Check sheet for the modelled part. Datum: model origin and axes. Units: mm. Face numbers are marked on the shaded views. A direction names the side the tool comes from. Round coordinates to 2 decimals unless told otherwise and drop trailing zeros. Order: outer loops, then holes, each group sorted by start corner. A loop starts at its lowest first (then second) coordinate and runs counter-clockwise, first axis right, second up. Notation, with made-up numbers: (67.25, 30) -> (111.25, 30) arc R20 cw to (111.25, 53) -> close; hole circle Ø6 at (11, 14.5). An arc over 180 degrees is marked (long way). Use CSV: the item, a comma, the result in double quotes.
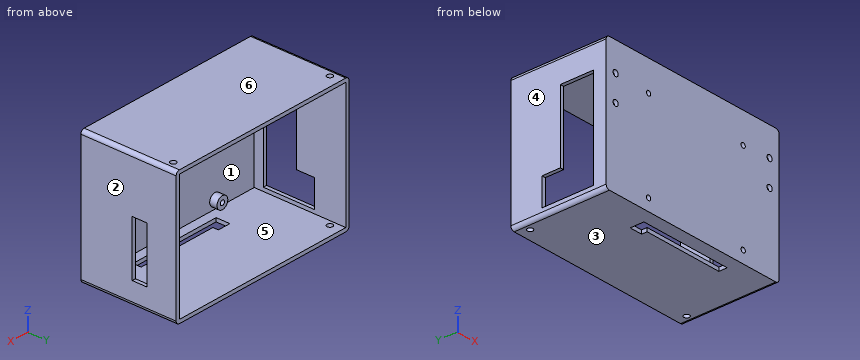
Autodesk Inventor part; units mm, degrees
ref_plane "YZ Plane" through (0, 0, 0) normal (1, 0, 0) x (0, 1, 0)
ref_plane "XZ Plane" through (0, 0, 0) normal (0, 1, 0) x (-1, 0, 0)
ref_plane "XY Plane" through (0, 0, 0) normal (0, 0, 1) x (1, 0, 0)
sketch "Náčrt1" plane through (0, 0, 0) normal (0, 1, 0) x (-1, 0, 0)
  line L0 (0, 0) -> (-106, 0)
  line L1 (-106, 0) -> (-106, -62)
  line L2 (-106, -62) -> (0, -62)
  line L3 (0, -62) -> (0, 0)
  line L4 (-104, -2) -> (-2, -2)
  line L5 (-2, -2) -> (-2, -60)
  line L6 (-2, -60) -> (-104, -60)
  line L7 (-104, -60) -> (-104, -2)
  line L8 (-5.8, 0) -> (-5.8, -18) construction
  circle A0 centre (-5.8, -19.6) radius 1.6
  line L9 (0, -19.6) -> (-4.2, -19.6) construction
  line L10 (-7.4, 0) -> (-7.4, -5.6) construction
  circle A1 centre (-5.8, -5.6) radius 1.6
  line L11 (0, -7.2) -> (-5.8, -7.2) construction
  line L12 (-53, 11.0609) -> (-53, -73.3805) construction
  line L13 (-100.2, 0) -> (-100.2, -18) construction
  circle A2 centre (-100.2, -19.6) radius 1.6
  line L14 (-106, -19.6) -> (-101.8, -19.6) construction
  line L15 (-98.6, 0) -> (-98.6, -5.6) construction
  circle A3 centre (-100.2, -5.6) radius 1.6
  line L16 (-106, -7.2) -> (-100.2, -7.2) construction
  dimension "d0" = 62
  dimension "d1" = 106
  dimension "d2" = 2
  dimension "d8" = 18
  dimension "d9" = 4.2
  dimension "d10" = 3.2
  dimension "d13" = 5.8
  dimension "d14" = 5.6
  dimension "d15" = 3.2
extrude "Vysunutí1" add sketch "Náčrt1" along normal blind 2 contours L4 L5 L6 L7 | A0 | A1 | A2 | A3
extrude "Vysunutí2" add sketch "Náčrt1" along normal blind 52 contours L3 L2 L1 L0
extrude "Vysunutí3" cut sketch "Náčrt1" along normal blind 2 contours A0 | A1 | A2 | A3
sketch "Náčrt2" plane through (0, 2, 0) normal (0, 1, 0) x (1, 0, 0)
  circle A0 centre (84, 55.5) radius 1.3
  line L0 (2, 60) -> (104, 60)
  circle A1 centre (26, 55.5) radius 1.3
  line L1 (2, 2) -> (2, 60)
  circle A2 centre (26, 6.5) radius 1.3
  circle A3 centre (84, 6.5) radius 1.3
  line L2 (104, 2) -> (2, 2)
  circle A4 centre (26, 6.5) radius 3.3
  circle A5 centre (26, 55.5) radius 3.3
  circle A6 centre (84, 55.5) radius 3.3
  circle A7 centre (84, 6.5) radius 3.3
  point P0 (0, 0)
  dimension "d19" = 4.5
  dimension "d20" = 2.6
  dimension "d21" = 2.6
  dimension "d22" = 58
  dimension "d23" = 24
  dimension "d24" = 4.5
  dimension "d25" = 2.6
  dimension "d26" = 24
  dimension "d27" = 2.6
  dimension "d28" = 58
  dimension "d29" = 4.5
  dimension "d30" = 4.5
  dimension "d31" = 49
  dimension "d32" = 2
  dimension "d33" = 2
  dimension "d34" = 2
  dimension "d35" = 2
extrude "Vysunutí4" add sketch "Náčrt2" along normal blind 4
extrude "Vysunutí5" cut sketch "Náčrt2" against normal blind 2 contours A0 | A1 | A2 | A3
sketch "Náčrt3" plane through (0, 0, -62) normal (-1, 0, 0) x (0, 0, 1)
  line L0 (4, 7) -> (58, 7)
  line L1 (58, 7) -> (58, 25)
  line L2 (58, 25) -> (4, 25)
  line L3 (4, 25) -> (4, 7)
  line L4 (9.8, 6) -> (3.2, 6)
  line L5 (2, 2) -> (2, 52)
  line L6 (60, 2) -> (60, 52)
  point P0 (62, 0)
  dimension "d40" = 1
  dimension "d41" = 54
  dimension "d42" = 18
  dimension "d43" = 2
  dimension "d44" = 2
extrude "Vysunutí6" cut sketch "Náčrt3" against normal blind 2
sketch "Náčrt4" plane through (106, 0, -62) normal (0, 0, -1) x (-1, 0, 0)
  line L0 (24, 7) -> (75, 7)
  line L1 (75, 7) -> (75, 11.5)
  line L2 (75, 11.5) -> (24, 11.5)
  line L3 (24, 11.5) -> (24, 7)
  line L4 (104, 2) -> (104, 52)
  line L5 (75, 11.5) -> (68, 11.5)
  line L6 (68, 11.5) -> (68, 14.5)
  line L7 (68, 14.5) -> (75, 14.5)
  line L8 (75, 14.5) -> (75, 11.5)
  line L9 (2, 2) -> (104, 2)
  point P0 (106, 0)
  point P1 (68, 11.5)
  dimension "d47" = 4.5
  dimension "d48" = 29
  dimension "d49" = 51
  dimension "d50" = 5
  dimension "d51" = 7.5
  dimension "d52" = 7
extrude "Vysunutí7" cut sketch "Náčrt4" against normal blind 2
sketch "Náčrt5" plane through (0, 0, 0) normal (0, -1, 0) x (1, 0, 0)
  line L0 (106, 0) -> (106, -62)
  line L1 (106, -2) -> (0, -2)
  line L2 (0, -2) -> (0, 10)
  line L3 (0, 10) -> (106, 10)
  line L4 (106, 10) -> (106, -2)
  line L5 (2, -2) -> (104, -2)
  line L6 (106, 10) -> (0, 10)
  line L7 (0, 10) -> (0, 8)
  line L8 (0, 8) -> (106, 8)
  line L9 (106, 8) -> (106, 10)
  line L10 (104, -60) -> (104, -2)
  line L11 (104, -2) -> (106, -2)
  line L12 (106, -2) -> (106, 10)
  line L13 (106, 10) -> (104, 10)
  line L14 (104, 10) -> (104, -2)
  line L15 (2, -2) -> (2, -60)
  line L16 (2, -2) -> (0, -2)
  line L17 (0, -2) -> (0, 10)
  line L18 (0, 10) -> (2, 10)
  line L19 (2, 10) -> (2, -2)
  point P0 (0, 0)
  point P1 (2, 8)
  point P2 (104, 8)
  dimension "d55" = 12
  dimension "d56" = 106
  dimension "d57" = 2
extrude "Vysunutí8" cut sketch "Náčrt5" against normal blind 52 contours L1 L19 L8 L14
extrude "Vysunutí9" add sketch "Náčrt5" against normal blind 2 contours L1 L19 L8 L14
extrude "Vysunutí10" add sketch "Náčrt5" against normal blind 52 contours L0 L1 L14 L8 L4 | L8 L14 L3 L4 | L8 L19 L3 L14 | L1 L2 L8 L19 | L8 L2 L3 L19
sketch "Náčrt6" plane through (0, 0, -62) normal (-1, 0, 0) x (0, 0, 1)
  line L0 (4, 25) -> (58, 25)
  line L1 (4, 25) -> (19, 25)
  line L2 (19, 25) -> (19, 35)
  line L3 (19, 35) -> (4, 35)
  line L4 (4, 35) -> (4, 25)
  point P0 (62, 0)
  dimension "d64" = 15
  dimension "d65" = 10
extrude "Vysunutí11" cut sketch "Náčrt6" against normal blind 4
fillet "Zaoblení1" radius 2 4 edges at (106, 26, -62) (0, 26, -62) (0, 26, 10) (106, 26, 10)
sketch "Náčrt7" plane through (2, 0, 10) normal (0, 0, 1) x (1, 0, 0)
  circle A0 centre (3, 46) radius 1.55
  line L0 (0, 52) -> (102, 52)
  line L1 (0, 0) -> (0, 52)
  circle A1 centre (99, 46) radius 1.55
  line L2 (102, 52) -> (102, 0)
  point P0 (-2, 0)
  dimension "d69" = 3.1
  dimension "d70" = 6
  dimension "d71" = 3
  dimension "d72" = 3.1
  dimension "d73" = 3
  dimension "d74" = 6
extrude "Vysunutí12" cut sketch "Náčrt7" against normal blind 400
sketch "Náčrt8" plane through (106, 0, 8) normal (1, 0, 0) x (0, 0, -1)
  line L0 (28, 36) -> (58, 36)
  line L1 (58, 36) -> (58, 28)
  line L2 (58, 28) -> (28, 28)
  line L3 (28, 28) -> (28, 36)
  line L4 (70, 0) -> (70, 52)
  line L5 (0, 0) -> (68, 0)
  point P0 (8, 0)
  dimension "d77" = 12
  dimension "d78" = 30
  dimension "d79" = 8
  dimension "d80" = 28
extrude "Vysunutí13" cut sketch "Náčrt8" against normal blind 52
equation "\"d21\" = d20"
equation "\"d24\" = d19"
equation "\"d25\" = d20"
equation "\"d26\" = d23"
equation "\"d27\" = d20"
equation "\"d28\" = d22"
equation "\"d29\" = d19"
equation "\"d30\" = d19"
equation "\"d33\" = d32"
equation "\"d34\" = d32"
equation "\"d35\" = d32"
properties part number "RPIholder"
Q1. Go/stop test with flat-tipped pins: pin 1 (3.5 mm diameter, centred on x = 5.8, z = -5.6, fed in from +Y); pin 2 (1.6 mm diameter, centred on x = 105, z = -34.5, fed in from -Y); pin 3 (5.5 mm diameter, centred on x = 27, z = -7.5, fed in from +Y). Record where each tip stops, or that it passes through.
Result sheet:
pin 1,"stops at y = 2"
pin 2,"stops at y = 0"
pin 3,"stops at y = 6"
Q2. Sectioned sample at C-C, the plane x = 77.5. Enter the section's corners in (y, z).
Result sheet:
outline,"(0, -62) -> (7, -62) -> (7, -60) -> (2, -60) -> (2, 8) -> (52, 8) -> (52, 10) -> (0, 10) -> close; (11.5, -62) -> (52, -62) -> (52, -60) -> (11.5, -60) -> close"
Q3. Access from +Z, -Z, +X, -X, +Y, -Y to the whole of each face (thin tool, end or side, straight path). Record for the marked faces 1 and 2.
Result sheet:
face 1,"+Y"
face 2,"+Z, -Z, +X, +Y, -Y"
Q4. Scan lines: L1, parallel to Z at x = 100.2, y = 0.7; L2, parallel to Z at x = 14.5, y = 33.5; L3, parallel to X at y = 43, z = -30. Record each from-to range of solid material in increasing order.
Result sheet:
L1,"z = -62 to -21.2, -18 to -7.2, -4 to 10"
L2,"z = -62 to -60, 8 to 10"
L3,"x = 0 to 2, 104 to 106"
Q5. Sectioned sample at B-B, the plane z = -36. Enter the section's corners in (x, y).
Result sheet:
outline,"(0, 0) -> (106, 0) -> (106, 28) -> (104, 28) -> (104, 2) -> (2, 2) -> (2, 7) -> (0, 7) -> close; (0, 25) -> (2, 25) -> (2, 52) -> (0, 52) -> close; (104, 36) -> (106, 36) -> (106, 52) -> (104, 52) -> close"
Q6. Sectioned sample at D-D, the plane y = 38.5. Enter the section's corners in (x, z).
Result sheet:
outline,"(0, -60) arc R2 ccw to (2, -62) -> (104, -62) arc R2 ccw to (106, -60) -> (106, 8) arc R2 ccw to (104, 10) -> (2, 10) arc R2 ccw to (0, 8) -> close; hole (2, -60) -> (104, -60) -> (104, 8) -> (2, 8) -> close"
Q7. Sectioned sample at A-A, the plane y = 30.5. Enter the section's corners in (x, z).
Result sheet:
outline,"(0, -60) arc R2 ccw to (2, -62) -> (104, -62) arc R2 ccw to (106, -60) -> (106, -50) -> (104, -50) -> (104, -60) -> (2, -60) -> (2, -58) -> (0, -58) -> close; (0, -43) -> (2, -43) -> (2, 8) -> (104, 8) -> (104, -20) -> (106, -20) -> (106, 8) arc R2 ccw to (104, 10) -> (2, 10) arc R2 ccw to (0, 8) -> close"
Q8. Mould release check, pull along Z, two halves, no side actions. Record for the marked faces 3, 4, 5 and 6: pulls with the +Z half, pulls with the -Z half, needs draft (parallel to the pull), parting line crosses it, or undercut.
Result sheet:
face 3,"pulls with the -Z half"
face 4,"needs draft"
face 5,"undercut"
face 6,"pulls with the +Z half"
